Can you work these out from the model? Positions are in its coordinate system, mm. Face numbers are marked on the shaded views. A direction names the side the tool comes from. Coordinates: 2 decimals unless noted, no trailing zeros. Loops run counter-clockwise (first coordinate to the right, second up) from the corner with the lowest first, then second, coordinate; pieces in that order, holes last. Notation, with made-up numbers: M 8,12 L 36,12 A25 ccw 36,38 Z; hole C 34,-7.5 d7. An arc over 180 degrees is marked long. Answer as a JSON object with one key per item and string values. Group by question number.
Item 1: Suppose I cut it at B-B (x = 33). Write out the boundary of the cut face in (y, z) (3 decimals), then the cut area to 3 significant figures.
Item 2: If I drill on line 1 (X direction, y = 41, z = -5.25) (3 decimals); line 2 (Z direction, x = 35, y = 38); line 3 (Z direction, x = 12, y = 40) (3 decimals), over which ranges is the centre line in solid material (lowest first)?
Item 3: Which directions (+Z, -Z, +X, -X, +Y, -Y) give clear straight access to the entire face, cutting with the end or side of a thin tool? Please do the marked faces 1 and 2.
Item 4: Suppose I cut it at D-D (y = 19). Write out the boundary of the cut face in (x, z) (3 decimals).
Item 5: I'm going to push a flat-ended pin straight in: pin 1 Ø2 at (y, z) = (10, -8.5) entering from -X (3 decimals). Where does the tip first touch, or does it pass through?
Item 6: Suppose I cut it at C-C (z = -10.75). Write out the boundary of the cut face in (x, y) (3 decimals), then the cut area to 3 significant figures.
Item 7: We'd pull the mould along Z, two halves only. Please class the marked faces 3, 4, 5 and 6: +Z half, -Z half, draft (parallel to the pull), parting line (faces both ways), or undercut.
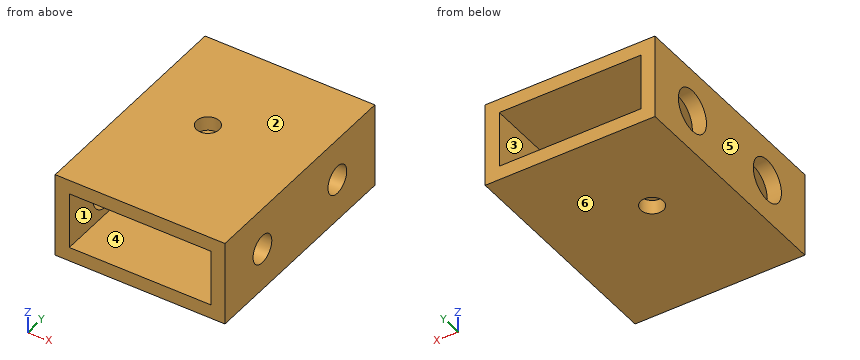
```python
from build123d import *

# Parameters (mm, degrees)
SKETCH1_W           = 38.1
SKETCH1_H           = 19.05
SKETCH1_W_2         = 31.75
SKETCH1_H_2         = 12.7
BOSS_EXTRUDE1_DEPTH = 50.8
SKETCH2_R           = 3.175
CUT_EXTRUDE1_DEPTH  = 39.1
SKETCH3_R           = 2.54
CUT_EXTRUDE2_DEPTH  = 20.05
CUT_EXTRUDE3_REACH  = 40.1
SKETCH4_R           = 4.7625


with BuildPart() as part:
    # Sketch1 → Boss-Extrude1 (new body)
    with BuildSketch(Plane(origin=(0, 0, 0), x_dir=(1, 0, 0), z_dir=(0, 1, 0))):
        with Locations((19.05, 9.525)):
            Rectangle(SKETCH1_W, SKETCH1_H)
        with Locations((19.05, 9.525)):
            Rectangle(SKETCH1_W_2, SKETCH1_H_2, mode=Mode.SUBTRACT)
    extrude(amount=BOSS_EXTRUDE1_DEPTH)

    # Sketch2 → Cut-Extrude1 (cut, through all)
    with BuildSketch(Plane(origin=(38.1, 0, 0), x_dir=(0, 0, -1), z_dir=(1, 0, 0))):
        with Locations((9.525, 38.1)):
            Circle(SKETCH2_R)
        with Locations((9.525, 12.7)):
            Circle(SKETCH2_R)
    extrude(amount=-CUT_EXTRUDE1_DEPTH, mode=Mode.SUBTRACT)

    # Sketch3 → Cut-Extrude2 (cut, through all)
    with BuildSketch(Plane.XY):
        with Locations((15.473378078, 28.395613607)):
            Circle(SKETCH3_R)
    extrude(amount=-CUT_EXTRUDE2_DEPTH, mode=Mode.SUBTRACT)

    # Sketch4 → Cut-Extrude3 (cut, up to next)
    with BuildSketch(Plane.ZY, mode=Mode.PRIVATE) as cut_extrude3_sk1:
        with Locations((-9.525, 12.7)):
            Circle(SKETCH4_R)
    cut_extrude3_tool1 = extrude(cut_extrude3_sk1.sketch, amount=-CUT_EXTRUDE3_REACH, mode=Mode.PRIVATE) & part.part
    add(cut_extrude3_tool1.solids().sort_by_distance((0, 12.7, -9.525))[0], mode=Mode.SUBTRACT)
    # Sketch4 → Cut-Extrude3 (cut, up to next)
    with BuildSketch(Plane.ZY, mode=Mode.PRIVATE) as cut_extrude3_sk2:
        with Locations((-9.525, 38.1)):
            Circle(SKETCH4_R)
    cut_extrude3_tool2 = extrude(cut_extrude3_sk2.sketch, amount=-CUT_EXTRUDE3_REACH, mode=Mode.PRIVATE) & part.part
    add(cut_extrude3_tool2.solids().sort_by_distance((0, 38.1, -9.525))[0], mode=Mode.SUBTRACT)


solid = part.part
```
From the geometry:
{
 "1": {"outline": "M 0,-19.05 L 50.8,-19.05 L 50.8,-15.875 L 0,-15.875 Z; M 0,-3.175 L 50.8,-3.175 L 50.8,0 L 0,0 Z", "area": "323 mm2"},
 "2": {"line 1": "0 to 3.175, 34.925 to 38.1", "line 2": "-19.05 to -12.7, -6.35 to 0", "line 3": "-19.05 to -15.875, -3.175 to 0"},
 "3": {"face 1": "+Y, -Y", "face 2": "+Z, +X, -X, +Y, -Y"},
 "4": {"outline": "M 0,-19.05 L 38.1,-19.05 L 38.1,0 L 0,0 Z; hole M 3.175,-15.875 L 34.925,-15.875 L 34.925,-3.175 L 3.175,-3.175 Z"},
 "5": {"pin 1": "x = 34.925"},
 "6": {"outline": "M 0,0 L 3.175,0 L 3.175,8.098 L 0,8.098 Z; M 0,17.302 L 3.175,17.302 L 3.175,33.498 L 0,33.498 Z; M 0,42.702 L 3.175,42.702 L 3.175,50.8 L 0,50.8 Z; M 34.925,0 L 38.1,0 L 38.1,9.771 L 34.925,9.771 Z; M 34.925,15.629 L 38.1,15.629 L 38.1,35.171 L 34.925,35.171 Z; M 34.925,41.029 L 38.1,41.029 L 38.1,50.8 L 34.925,50.8 Z", "area": "227 mm2"},
 "7": {"face 3": "undercut", "face 4": "undercut", "face 5": "draft", "face 6": "-Z half"}
}
